Here's how the part is built. I have some questions about the finished solid (model axes, mm). Face numbers are marked on the shaded views. Coordinates: 2 decimals unless noted, no trailing zeros. Write each loop counter-clockwise with the first axis right and the second up, starting at its lowest first coordinate (ties: lowest second). Pieces come first, ordered by that corner, then holes. Notation, with made-up numbers: (19.25, -23.75) -> (56.25, -23.75) arc R22 cw to (56.25, 8.25) -> close; hole circle Ø4 at (53, 58). An arc over 180 degrees is marked (long way). Use a Markdown table: item, result. Add a question column.
Item 1: If we mould it in two halves opening along Y, with no side actions, what happens to the marked faces 1, 2 and 3? For each: pulls with the +Y half, pulls with the -Y half, needs draft (parallel to the pull), parting line crosses it, or undercut.
Item 2: If I drill on line 1 along Y through (x, z) = (0, -8.5); line 2 along X through (y, z) = (-12.5, 40.5), over which ranges is the centre line in solid material (lowest first)? Write a range as from..to.
Item 3: Imagine slicing it at A-A, the plane x = 0. Write out the boundary of the cut face in (y, z).
Item 4: Will these pins go through, and if not, where does the flat tip stop? pin 1 Ø2 at (x, z) = (17.5, 5) entering from +Y; pin 2 Ø1 at (x, z) = (30.5, 21.5) entering from +Y; pin 3 Ø10 at (y, z) = (24, 42) entering from -X; pin 4 Ø10 at (y, z) = (3, 17) entering from -X.
Item 5: Imagine slicing it at C-C, the plane z = 34. Write out the boundary of the cut face in (x, y).
```python
from build123d import *

# Parameters (mm, degrees)
F0_R        = 64.282036
F0_R_2      = 56.51558
F1_DEPTH    = 52.07
F2_R        = 63.645379
F2_R_2      = 59.669369
F3_DEPTH    = 28.194
F1_FACE_R   = 64.282036
F1_FACE_R_2 = 56.51558
F4_DEPTH    = 25.4


with BuildPart() as f1:
    # F0 (on Top) → F1 (new body)
    with BuildSketch(Plane.XY):
        Circle(F0_R)
        Circle(F0_R_2, mode=Mode.SUBTRACT)
    extrude(amount=F1_DEPTH)

    # F2 (on Top) → F3 (join)
    with BuildSketch(Plane.XY):
        Circle(F2_R)
        Circle(F2_R_2, mode=Mode.SUBTRACT)
    extrude(amount=F3_DEPTH)

    # F1_face (on face) → F4 (join)
    with BuildSketch(Plane(origin=(0, 0, 0), x_dir=(1, 0, 0), z_dir=(0, 0, -1))):
        Circle(F1_FACE_R)
        Circle(F1_FACE_R_2, mode=Mode.SUBTRACT)
    extrude(amount=F4_DEPTH)


solid = f1.part
```
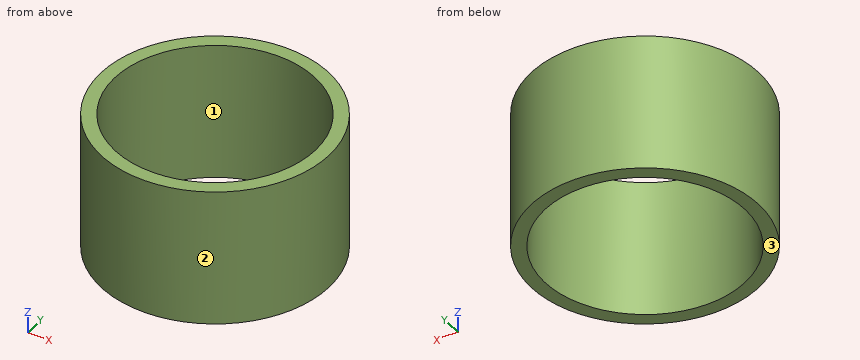
Ans:
| question | item | result |
|---|---|---|
| 1 | face 1 | undercut |
| 1 | face 2 | parting line crosses it |
| 1 | face 3 | needs draft |
| 2 | line 1 | y = -64.28..-56.52, 56.52..64.28 |
| 2 | line 2 | x = -63.05..-55.12, 55.12..63.05 |
| 3 | outline | (-64.28, -25.4) -> (-56.52, -25.4) -> (-56.52, 52.07) -> (-64.28, 52.07) -> close; (56.52, -25.4) -> (64.28, -25.4) -> (64.28, 52.07) -> (56.52, 52.07) -> close |
| 4 | pin 1 | stops at y = 62.13 |
| 4 | pin 2 | stops at y = 56.85 |
| 4 | pin 3 | stops at x = -61.41 |
| 4 | pin 4 | stops at x = -64.28 |
| 5 | outline | circle Ø128.56 at (0, 0); hole circle Ø113.03 at (0, 0) |
